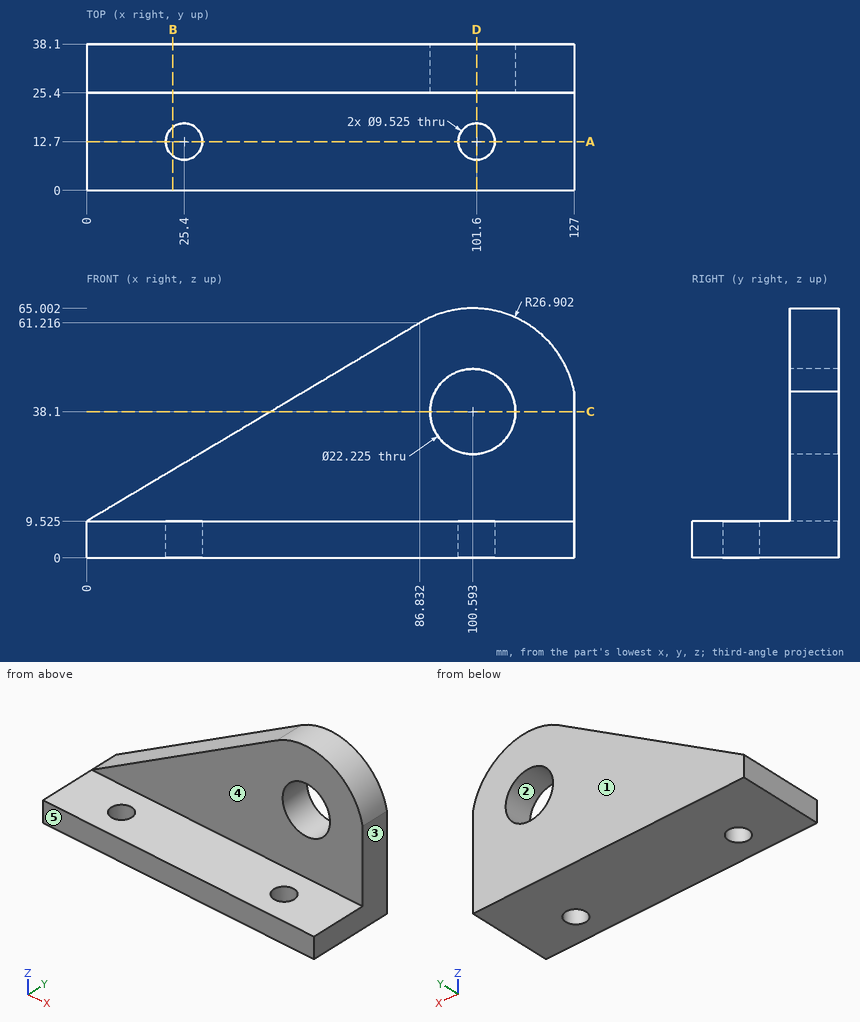
The drawing under review shows one solid part. Ordinate dimensions are in mm from its lowest x, y, z. A direction names the side the tool comes from. Round coordinates to 2 decimals unless told otherwise and drop trailing zeros. Order: outer loops, then holes, each group sorted by start corner. A loop starts at its lowest first (then second) coordinate and runs counter-clockwise, first axis right, second up. Notation, with made-up numbers: (23.5, 18.5) -> (67.5, 18.5) arc R4 ccw to (67.5, 23.5) -> close; hole circle Ø9 at (-22, 14). An arc over 180 degrees is marked (long way). Use a Markdown table: item, result.
Q1. We need section C-C on z = 38.1. Write out the cut boundary in (x, y) (1 decimal), then the cut area to 3 significant figures.
Values:
| item | result |
|---|---|
| outline | (48, 25.4) -> (89.5, 25.4) -> (89.5, 38.1) -> (48, 38.1) -> close; (111.7, 25.4) -> (127, 25.4) -> (127, 38.1) -> (111.7, 38.1) -> close |
| area | 721 mm^2 |
Q2. Clearance check with flat-ended pins moving along their axes: P1, Ø8, axis at y = 17.5, z = 28, coming from the -X side; P2, Ø10, axis at x = 27, y = 33.5, coming from the +Z side (1 decimal); P3, Ø1, axis at x = 74.5, y = 12.5, coming from the +Z side (3 decimals). State where each tip first meets the part, or that it passes through.
Values:
| item | result |
|---|---|
| P1 | passes through |
| P2 | stops at z = 28.6 |
| P3 | stops at z = 9.525 |
Q3. Tool access review of the marked faces 4 and 5: name each direction out of +Z, -Z, +X, -X, +Y, -Y from which nothing blocks a thin tool from reaching the whole face with its end or side.
Values:
| item | result |
|---|---|
| face 4 | +Z, +X, -X, -Y |
| face 5 | +Z, -Z, +X, -X, -Y |
Q4. Mouldability with a two-part tool opening along X and no side actions: class the marked faces 1, 2 and 3 as +X half, -X half, draft (parallel to the pull), parting line (faces both ways), or undercut.
Values:
| item | result |
|---|---|
| face 1 | draft |
| face 2 | undercut |
| face 3 | +X half |
Q5. We need section D-D on x = 101.6. Write out the cut boundary in (y, z) (1 decimal).
Values:
| item | result |
|---|---|
| outline | (0, 0) -> (7.9, 0) -> (7.9, 9.5) -> (0, 9.5) -> close; (17.5, 0) -> (38.1, 0) -> (38.1, 27) -> (25.4, 27) -> (25.4, 9.5) -> (17.5, 9.5) -> close; (25.4, 49.2) -> (38.1, 49.2) -> (38.1, 65) -> (25.4, 65) -> close |
Q6. We need section A-A on y = 12.7. Write out the cut boundary in (x, z) (1 decimal), then the cut area to 3 significant figures.
Values:
| item | result |
|---|---|
| outline | (0, 0) -> (20.6, 0) -> (20.6, 9.5) -> (0, 9.5) -> close; (30.2, 0) -> (96.8, 0) -> (96.8, 9.5) -> (30.2, 9.5) -> close; (106.4, 0) -> (127, 0) -> (127, 9.5) -> (106.4, 9.5) -> close |
| area | 1,030 mm^2 |
Q7. We need section B-B on x = 22.5. Write out the cut boundary in (y, z) (1 decimal), then the cut area to 3 significant figures.
Values:
| item | result |
|---|---|
| outline | (0, 0) -> (8.9, 0) -> (8.9, 9.5) -> (0, 9.5) -> close; (16.5, 0) -> (38.1, 0) -> (38.1, 22.9) -> (25.4, 22.9) -> (25.4, 9.5) -> (16.5, 9.5) -> close |
| area | 461 mm^2 |
Q8. For line 1 (Y direction, x = 25, z = 5) (1 decimal); line 2 (X direction, y = 12, z = 2); line 3 (Y direction, x = 101.6, z = 7), list the stretches that pass through material, from the lowest coordinate up.
Values:
| item | result |
|---|---|
| line 1 | y = 0 to 8, 17.4 to 38.1 |
| line 2 | x = 0 to 20.69, 30.11 to 96.89, 106.31 to 127 |
| line 3 | y = 0 to 7.94, 17.46 to 38.1 |
